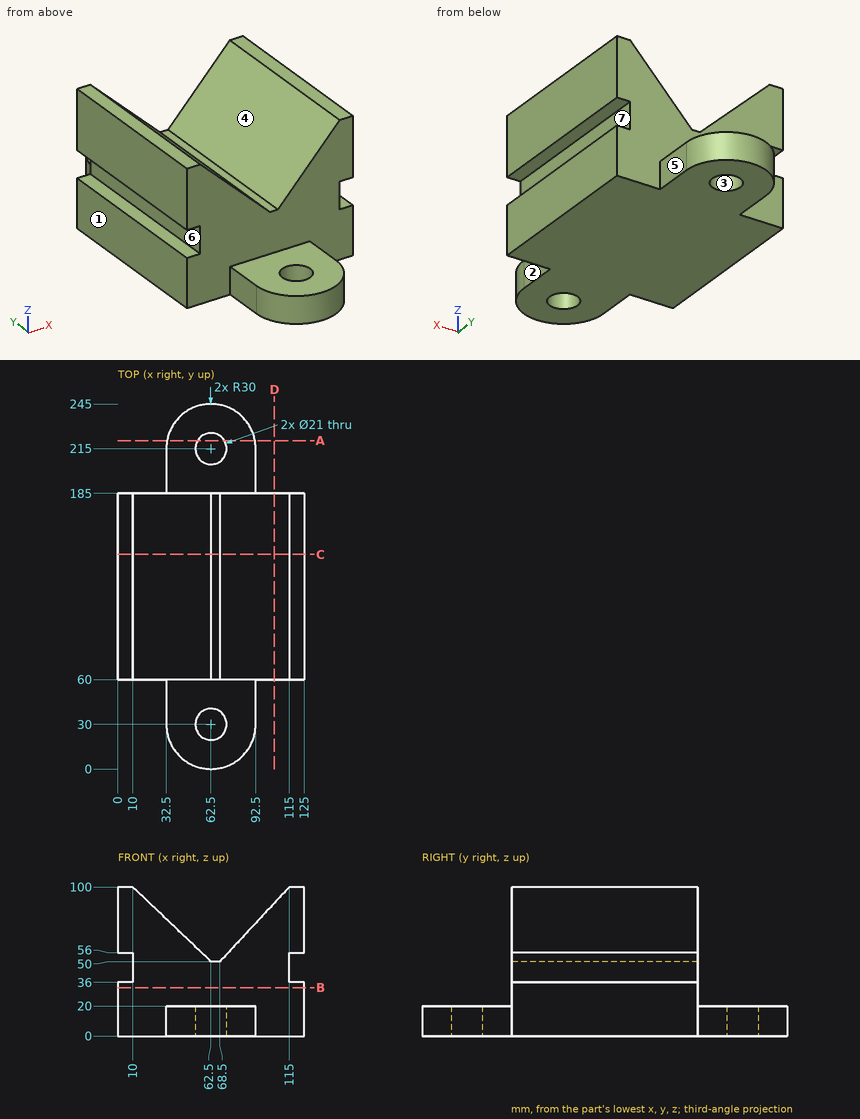
Drawing for the job (mm, zero at the part's lowest x, y, z). A direction names the side the tool comes from. Give positions to 0.01 mm unless a question says otherwise; leave off trailing zeros. Write each loop counter-clockwise with the first axis right and the second up, starting at its lowest first coordinate (ties: lowest second). Pieces come first, ordered by that corner, then holes. Notation, with made-up numbers: M 19,-10.5 L 72,-10.5 A11 ccw 72,-4.5 Z; hole C 61,-35 d6. An arc over 180 degrees is marked long. Use CSV: the item, a comma, the result in double quotes.
Item 1: Drill centre lines: probe 1 along Y at (x, z) = (62.5, 10.75); probe 2 along Y at (x, z) = (64.5, 9); probe 3 along Y at (x, z) = (19, 8.5). Where is each one in solid material? Low to high.
Taken from the geometry:
probe 1,"y = 0 to 19.5, 40.5 to 204.5, 225.5 to 245"
probe 2,"y = 0.07 to 19.69, 40.31 to 204.69, 225.31 to 244.93"
probe 3,"y = 60 to 185"
Item 2: Slice it at C-C on y = 144. Write the cut outline in (x, z), plus the area to 4 significant figures.
Taken from the geometry:
outline,"M 0,0 L 125,0 L 125,36 L 115,36 L 115,56 L 125,56 L 125,100 L 115,100 L 68.5,50 L 62.5,50 L 10,100 L 0,100 L 0,56 L 10,56 L 10,36 L 0,36 Z"
area,"9,325 mm²"
Item 3: Slice it at A-A on y = 220.5. Write the cut outline in (x, z), plus the area to 3 significant figures.
Taken from the geometry:
outline,"M 33.01,0 L 53.56,0 L 53.56,20 L 33.01,20 Z; M 71.44,0 L 91.99,0 L 91.99,20 L 71.44,20 Z"
area,"822 mm²"
Item 4: Slice it at D-D on x = 105. Write the cut outline in (y, z), plus the area to 3 significant figures.
Taken from the geometry:
outline,"M 60,0 L 185,0 L 185,89.25 L 60,89.25 Z"
area,"11,200 mm²"
Item 5: Slice it at B-B on z = 32.5. Write the cut outline in (x, y).
Taken from the geometry:
outline,"M 0,60 L 125,60 L 125,185 L 0,185 Z"
Item 6: Pin check, flat tips, straight feed: P1, Ø5, axis at x = 32.5, z = 16, coming from the +Y side; P2, Ø12, axis at x = 31.5, z = 69.5, coming from the +Y side; P3, Ø5, axis at y = 168.5, z = 52.5, coming from the -X side. Stop position of each tip, or through.
Taken from the geometry:
P1,"stops at y = 226.99"
P2,"stops at y = 185"
P3,"stops at x = 10"
Item 7: Which spindle directions (+Z, -Z, +X, -X, +Y, -Y) get a long thin tool onto all of the face, cutting with end or side? Do the marked faces 4, 5, 6 and 7. Say none if no direction does.
Taken from the geometry:
face 4,"+Z, +Y, -Y"
face 5,"+Z, -Z, +X, +Y"
face 6,"-X, +Y, -Y"
face 7,"+X, +Y, -Y"
Item 8: Pull direction X, two halves, no side cores. Call the marked faces 1, 2 and 3: +X half, -X half, draft (parallel to the pull), parting line (faces both ways), or undercut.
Taken from the geometry:
face 1,"-X half"
face 2,"+X half"
face 3,"undercut"
